Part model, mm, in its own coordinate system. A direction names the side the tool comes from. Coordinates: 2 decimals unless noted, no trailing zeros. Loops run counter-clockwise (first coordinate to the right, second up) from the corner with the lowest first, then second, coordinate; pieces in that order, holes last.
```python
from build123d import *

# Parameters (mm, degrees)
SKETCH1_W                         = 59
SKETCH1_H                         = 120
SKETCH1_R                         = 10.5
BOSS_EXTRUDE1_DEPTH               = 12
BOSS_EXTRUDE2_DEPTH               = 12
SKETCH9_W                         = 48
SKETCH9_H                         = 133
BOSS_EXTRUDE3_DEPTH               = 12
SKETCH11_W                        = 10
SKETCH11_H                        = 160
BOSS_EXTRUDE4_DEPTH               = 12
CHAMFER1_SIZE                     = 10
CHAMFER2_SIZE                     = 10
F_10_0_10_DIAMETER_HOLE1_D        = 10
F_6_0_6_DIAMETER_HOLE1_AT_2_COUNT = 2
F_6_0_6_DIAMETER_HOLE1_AT_2_PITCH = 91
F_6_0_6_DIAMETER_HOLE3_D          = 6
F_6_0_6_DIAMETER_HOLE3_DEPTH      = 20
F_6_0_6_DIAMETER_HOLE3_TIP        = 1.802581857
F_6_0_6_DIAMETER_HOLE4_D          = 6
F_6_0_6_DIAMETER_HOLE5_D          = 6
F_6_0_6_DIAMETER_HOLE5_DEPTH      = 20
F_6_0_6_DIAMETER_HOLE5_TIP        = 1.802581857
HOLE2_D                           = 12
HOLE2_DEPTH                       = 6
SKETCH27_R                        = 12
CUT_EXTRUDE1_DEPTH                = 8


with BuildPart() as part:
    # Sketch1 → Boss-Extrude1 (new body)
    with BuildSketch(Plane(origin=(0, 0, 0), x_dir=(0, 0, -1), z_dir=(1, 0, 0))):
        Rectangle(SKETCH1_W, SKETCH1_H)
        Circle(SKETCH1_R, mode=Mode.SUBTRACT)
    extrude(amount=BOSS_EXTRUDE1_DEPTH)

    # Sketch8 → Boss-Extrude2 (add)
    with BuildSketch(Plane.ZY):
        Polygon((42.5, 18), (42.5, -12), (54.5, -12), (54.5, 60), (29.5, 60), (29.5, -60), (30.5, -60), (30.5, 18), align=None)
    extrude(amount=-BOSS_EXTRUDE2_DEPTH)

    # Sketch9 → Boss-Extrude3 (add)
    with BuildSketch(Plane.ZY):
        with Locations((6.5, -126.5)):
            Rectangle(SKETCH9_W, SKETCH9_H)
    extrude(amount=-BOSS_EXTRUDE3_DEPTH)

    # Sketch11 → Boss-Extrude4 (add)
    with BuildSketch(Plane(origin=(12, 0, 0), x_dir=(0, 0, -1), z_dir=(1, 0, 0))):
        with Locations((34.5, -20)):
            Rectangle(SKETCH11_W, SKETCH11_H)
    extrude(amount=-BOSS_EXTRUDE4_DEPTH)

    # Chamfer1
    chamfer1_edges = [part.edges().sort_by_distance(p)[0] for p in [
        (6, 60, 54.5),
        (6, -12, 54.5),
        (6, 60, -39.5),
    ]]
    chamfer(chamfer1_edges, length=CHAMFER1_SIZE)

    # Chamfer2
    chamfer2_edges = [part.edges().sort_by_distance(p)[0] for p in [
        (6, -100, -39.5),
    ]]
    chamfer(chamfer2_edges, length=CHAMFER2_SIZE - 0.0001)  # a hair under: the kernel refuses the full size

    # Ø10.0 (10) Diameter Hole1 (through all)
    with Locations(Plane(origin=(12, 0, 0), x_dir=(0, 0, -1), z_dir=(1, 0, 0))):
        with Locations((-18.5, -169), (5.5, -169), (-18.5, -78), (5.5, -78)):
            Hole(F_10_0_10_DIAMETER_HOLE1_D / 2)

    # Sketch15 → Ø6.0 (6) Diameter Hole1 (revolve, cut)
    with BuildSketch(Plane(origin=(6, -169, -17.5), x_dir=(0, 1, 0), z_dir=(1, 0, 0))):
        Polygon((0, 0), (0, 21.802581857), (3, 20), (3, 0), align=None)
    f_6_0_6_diameter_hole1 = revolve(axis=Axis((6, -169, -23.85), (0, 0, 1)), mode=Mode.SUBTRACT)

    # Ø6.0 (6) Diameter Hole1 at 2: Ø6.0 (6) Diameter Hole1 ×2
    with Locations(*[(0, i * F_6_0_6_DIAMETER_HOLE1_AT_2_PITCH, 0) for i in range(1, F_6_0_6_DIAMETER_HOLE1_AT_2_COUNT)]):
        add(f_6_0_6_diameter_hole1, mode=Mode.SUBTRACT)

    # Ø6.0 (6) Diameter Hole3
    with Locations(Plane(origin=(0, 0, -39.5), x_dir=(-1, 0, 0), z_dir=(0, 0, -1))):
        with Locations((-6, -78)):
            Hole(F_6_0_6_DIAMETER_HOLE3_D / 2, depth=F_6_0_6_DIAMETER_HOLE3_DEPTH)
            with Locations((0, 0, -(F_6_0_6_DIAMETER_HOLE3_DEPTH + F_6_0_6_DIAMETER_HOLE3_TIP / 2))):  # 118° drill point
                Cone(0, F_6_0_6_DIAMETER_HOLE3_D / 2, F_6_0_6_DIAMETER_HOLE3_TIP, mode=Mode.SUBTRACT)

    # Ø6.0 (6) Diameter Hole4 (through all)
    with Locations(Plane(origin=(12, 0, 0), x_dir=(0, 0, -1), z_dir=(1, 0, 0))):
        with Locations((-36.5, 36)):
            Hole(F_6_0_6_DIAMETER_HOLE4_D / 2)

    # Ø6.0 (6) Diameter Hole5
    with Locations(Plane.XY.offset(30.5)):
        with Locations((6, -78), (6, -169)):
            Hole(F_6_0_6_DIAMETER_HOLE5_D / 2, depth=F_6_0_6_DIAMETER_HOLE5_DEPTH)
            with Locations((0, 0, -(F_6_0_6_DIAMETER_HOLE5_DEPTH + F_6_0_6_DIAMETER_HOLE5_TIP / 2))):  # 118° drill point
                Cone(0, F_6_0_6_DIAMETER_HOLE5_D / 2, F_6_0_6_DIAMETER_HOLE5_TIP, mode=Mode.SUBTRACT)

    # Hole2
    with Locations(Plane(origin=(12, 0, 0), x_dir=(0, 0, -1), z_dir=(1, 0, 0))):
        with Locations((0, -45), (0, 45)):
            Hole(HOLE2_D / 2, depth=HOLE2_DEPTH)

    # Sketch27 → Cut-Extrude1 (cut)
    with BuildSketch(Plane(origin=(12, 0, 0), x_dir=(0, 0, -1), z_dir=(1, 0, 0))):
        Circle(SKETCH27_R)
    extrude(amount=-CUT_EXTRUDE1_DEPTH, mode=Mode.SUBTRACT)


solid = part.part
```
Q1. Saw through at B-B (y = 45). List the corners of the cut face in (x, z), plus the area to 3 significant figures.
Q2. Tool access for faces 5 (the cylindrical face through (6, -172, -14)), 6 (the flat face through (6, -60, -24)), 7 (the cylindrical face through (8.4, -170.8, 12.5)): list every direction of +Z, -Z, +X, -X, +Y, -Y with a clear straight run to the whole face (end or side of a thin tool).
Q3. Saw through at A-A (y = -45). List the corners of the cut face in (x, z).
Q4. Probe line 1 (Y direction, x = 6, z = 28.75); line 2 (Z direction, x = 2.25, y = 1); line 3 (Z direction, x = 4.5, y = -81). List the from-to ranges inside material, lowest first.
Q5. Drop flat-ended pins along their axis: P1, Ø7, axis at y = 45, z = 0, coming from the +X side; P2, Ø3.5, axis at x = 6, y = -78, coming from the -Z side; P3, Ø5.5, axis at x = 6, y = -169, coming from the -Z side. Give the stop position or say it passes through.
Q6. Saw through at C-C (y = -117). List the corners of the cut face in (x, z), plus the area to 3 significant figures.
Q7. Mould opens along Z. For faces 1 (the cylindrical face through (8.958, -50.857, -1.301)), 2 (the cylindrical face through (5.916, -74.621, 14.815)), 3 (the flat face through (5.9, 54.9, 49.6)), 4 (the flat face through (6.1, 55.1, -34.4)) say: released by +Z, released by -Z, zero draft, split by the parting line, or undercut.
Checked values:
1. outline: (0, -39.5) - (12, -39.5) - (12, -6) - (6, -6) - (6, 6) - (12, 6) - (12, 54.5) - (0, 54.5) - close
1. area: 1,060 mm2
2. face 5: -Z
2. face 6: +X, -X, -Y
2. face 7: +Z
3. outline: (0, -39.5) - (12, -39.5) - (12, -6) - (6, -6) - (6, 6) - (12, 6) - (12, 30.5) - (0, 30.5) - close
4. line 1: y = -193 to -172, -166 to -81, -75 to 60
4. line 2: z = -39.5 to -10.45, 10.45 to 30.5, 42.5 to 54.5
4. line 3: z = -39.5 to -29.5, -17.5 to -9.5, -1.5 to 14.5, 22.5 to 30.5
5. P1: stops at x = 6
5. P2: stops at z = 3.25
5. P3: stops at z = 2.65
6. outline: (0, -17.5) - (12, -17.5) - (12, 30.5) - (0, 30.5) - close
6. area: 576 mm2
7. face 1: undercut
7. face 2: undercut
7. face 3: released by +Z
7. face 4: released by -Z
